Geometry: final body of the model. Coordinates: model frame, mm. Face numbers are marked on the shaded views. A direction names the side the tool comes from. Round coordinates to 2 decimals unless told otherwise and drop trailing zeros. Loops run counter-clockwise (first coordinate to the right, second up) from the corner with the lowest first, then second, coordinate; pieces in that order, holes last. Notation, with made-up numbers: (-32, 19.25) - (-3, 19.25) arc R9 ccw to (-3, 36.25) - close; hole circle Ø2 at (-6, 72). An arc over 180 degrees is marked (long way). Answer as CSV lines item,"result".
from build123d import *

# Parameters (mm, degrees)
F1_DEPTH = 10
F2_W     = 5
F2_H     = 5
F3_DEPTH = 10
F4_R     = 1.65
F5_DEPTH = 10.001
F6_R     = 5


with BuildPart() as f1:
    # F0 (on Top) → F1 (new body)
    with BuildSketch(Plane.XY):
        Polygon((25, 10), (-25, 10), (-25, -10), (-12, -10), (-12, 0), (12, 0), (12, -10), (25, -10), align=None)
    extrude(amount=F1_DEPTH)

    # F2 (on face) → F3 (cut)
    with BuildSketch(Plane.XY.offset(10)):
        with Locations((-18, -5)):
            Rectangle(F2_W, F2_H)
        with BuildLine():
            Line((-20.5, -7.5), (-20.5, -2.5))
            ThreePointArc((-20.5, -2.5), (-23, -5), (-20.5, -7.5))
        make_face()
        with BuildLine():
            ThreePointArc((-15.5, -7.5), (-13, -5), (-15.5, -2.5))
            Line((-15.5, -2.5), (-15.5, -7.5))
        make_face()
        with Locations((18, -5)):
            Rectangle(F2_W, F2_H)
        with BuildLine():
            Line((15.5, -7.5), (15.5, -2.5))
            ThreePointArc((15.5, -2.5), (13, -5), (15.5, -7.5))
        make_face()
        with BuildLine():
            ThreePointArc((20.5, -7.5), (23, -5), (20.5, -2.5))
            Line((20.5, -2.5), (20.5, -7.5))
        make_face()
    extrude(amount=-F3_DEPTH, mode=Mode.SUBTRACT)

    # F4 (on face) → F5 (cut, through all)
    with BuildSketch(Plane.XZ):
        with Locations((-7.5, 5)):
            Circle(F4_R)
        with Locations((7.5, 5)):
            Circle(F4_R)
    extrude(amount=-F5_DEPTH, mode=Mode.SUBTRACT)

    # F6
    f6_edges = [f1.edges().sort_by_distance(p)[0] for p in [
        (-25, -10, 5),
        (-12, -10, 5),
        (12, -10, 5),
        (25, -10, 5),
        (25, 10, 5),
        (-25, 10, 5),
    ]]
    fillet(f6_edges, radius=F6_R)


solid = f1.part
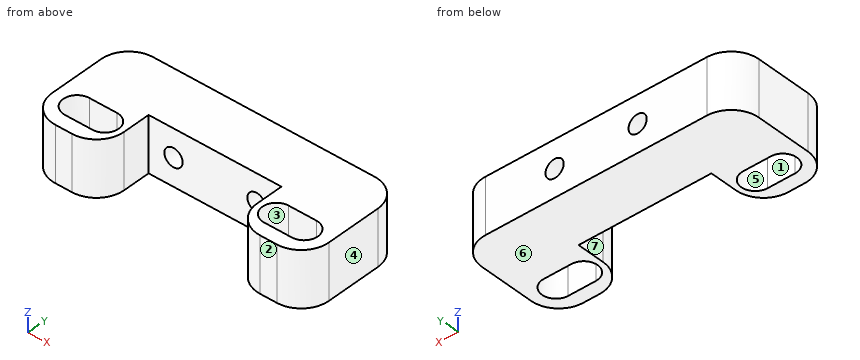
(1) Section B-B (x = 19). Output: boundary loops of the cut face in (y, z), and give its area (3 significant figures).
Findings below:
outline,"(-10, 0) - (-7.5, 0) - (-7.5, 10) - (-10, 10) - close; (-2.5, 0) - (10, 0) - (10, 10) - (-2.5, 10) - close"
area,"150 mm2"
(2) Draft query along Y for the marked faces 1, 2, 3 and 4. Return one class per face: pulls with the +Y half, pulls with the -Y half, needs draft (parallel to the pull), parting line crosses it, or undercut.
Findings below:
face 1,"undercut"
face 2,"pulls with the -Y half"
face 3,"undercut"
face 4,"needs draft"
(3) Section A-A (y = -1). Output: boundary loops of the cut face in (x, z).
Findings below:
outline,"(-25, 0) - (-12, 0) - (-12, 10) - (-25, 10) - close; (12, 0) - (25, 0) - (25, 10) - (12, 10) - close"
(4) Pin query (flat end, axial travel): P1, Ø4, axis at x = 7.5, z = 5, coming from the -Y side. Return the tip coordinate at first contact, or that it passes through.
Findings below:
P1,"y = 0"
(5) Section D-D (y = -3.25). Output: boundary loops of the cut face in (x, z), and give its area (3 significant figures).
Findings below:
outline,"(-25, 0) - (-22.29, 0) - (-22.29, 10) - (-25, 10) - close; (-13.71, 0) - (-12, 0) - (-12, 10) - (-13.71, 10) - close; (12, 0) - (13.71, 0) - (13.71, 10) - (12, 10) - close; (22.29, 0) - (25, 0) - (25, 10) - (22.29, 10) - close"
area,"88.6 mm2"
(6) Material intervals for line 1 along Z through (x, y) = (-7.5, 8.25); line 2 along X through (y, z) = (8, 5.25); line 3 along X through (y, z) = (-7.25, 6.5), sorted ascending.
Findings below:
line 1,"0 to 3.35, 6.65 to 10"
line 2,"-24 to -9.13, -5.87 to 5.87, 9.13 to 24"
line 3,"-24.47 to -21.59, -14.41 to -12.53, 12.53 to 14.41, 21.59 to 24.47"
(7) Access query for the marked faces 5, 6 and 7. Directions: +Z, -Z, +X, -X, +Y, -Y. A direction counts if a zero-diameter tool reaches every point of the face in a straight line with its end or side. Return the directions, or none.
Findings below:
face 5,"+Z, -Z"
face 6,"-Z, +X, -X, +Y, -Y"
face 7,"+Z, -Z, -Y"
(8) Section C-C (z = 9). Output: boundary loops of the cut face in (x, y).
Findings below:
outline,"(-25, -5) arc R5 ccw to (-20, -10) - (-17, -10) arc R5 ccw to (-12, -5) - (-12, 0) - (12, 0) - (12, -5) arc R5 ccw to (17, -10) - (20, -10) arc R5 ccw to (25, -5) - (25, 5) arc R5 ccw to (20, 10) - (-20, 10) arc R5 ccw to (-25, 5) - close; hole (-20.5, -7.5) - (-15.5, -7.5) arc R2.5 ccw to (-15.5, -2.5) - (-20.5, -2.5) arc R2.5 ccw to start; hole (15.5, -7.5) - (20.5, -7.5) arc R2.5 ccw to (20.5, -2.5) - (15.5, -2.5) arc R2.5 ccw to start"
